from build123d import *

# Parameters (mm, degrees)
SZKIC2_R                   = 1.75
WYTNIJ_WYCI_GNI_CIE1_DEPTH = 15.013168353
SZKIC4_R                   = 3
WYTNIJ_WYCI_GNI_CIE2_DEPTH = 4
SFAZOWANIE1_SIZE           = 1


with BuildPart() as part:
    # Szkic1 → Obrót1 (revolve)
    with BuildSketch(Plane.XY):
        Polygon((-272.858046523, 75.009269975), (-280.358046523, 75.009269975), (-280.358046523, 68.009269975), (-286.871214876, 68.009269975), (-286.871214876, 85.009269975), (-285.871214876, 86.009269975), (-272.858046523, 86.009269975), align=None)
    revolve(axis=Axis((-268.908046523, 1.009269975, 0), (-1, 0, 0)))

    # Szkic2 → Wytnij-wyciągnięcie1 (cut, through all)
    with BuildSketch(Plane.ZY.offset(286.871214876)):
        with Locations((79.5, 1.009269975)):
            Circle(SZKIC2_R)
        with Locations((56.214989104, -55.20571913)):
            Circle(SZKIC2_R)
        with Locations((0, -78.490730025)):
            Circle(SZKIC2_R)
        with Locations((-56.214989104, -55.20571913)):
            Circle(SZKIC2_R)
        with Locations((-79.5, 1.009269975)):
            Circle(SZKIC2_R)
        with Locations((-56.214989104, 57.224259079)):
            Circle(SZKIC2_R)
        with Locations((0, 80.509269975)):
            Circle(SZKIC2_R)
        with Locations((56.214989104, 57.224259079)):
            Circle(SZKIC2_R)
    extrude(amount=-WYTNIJ_WYCI_GNI_CIE1_DEPTH, mode=Mode.SUBTRACT)

    # Szkic4 → Wytnij-wyciągnięcie2 (cut)
    with BuildSketch(Plane.ZY.offset(286.871214876)):
        with Locations((79.5, 1.009269975)):
            Circle(SZKIC4_R)
        with Locations((56.214989104, -55.20571913)):
            Circle(SZKIC4_R)
        with Locations((0, -78.490730025)):
            Circle(SZKIC4_R)
        with Locations((-56.214989104, -55.20571913)):
            Circle(SZKIC4_R)
        with Locations((-79.5, 1.009269975)):
            Circle(SZKIC4_R)
        with Locations((-56.214989104, 57.224259079)):
            Circle(SZKIC4_R)
        with Locations((0, 80.509269975)):
            Circle(SZKIC4_R)
        with Locations((56.214989104, 57.224259079)):
            Circle(SZKIC4_R)
    extrude(amount=-WYTNIJ_WYCI_GNI_CIE2_DEPTH, mode=Mode.SUBTRACT)

    # Sfazowanie1
    sfazowanie1_edges = [part.edges().sort_by_distance(p)[0] for p in [
        (-280.358046523, -65.990730025, 0),
    ]]
    chamfer(sfazowanie1_edges, length=SFAZOWANIE1_SIZE)


solid = part.part
The listing builds one solid part. Answer for the finished solid, in the listing's coordinates (mm). A direction names the side the tool comes from. Give positions to 0.01 mm unless a question says otherwise; leave off trailing zeros.
Item 1: Each of these flat-tipped pins is pushed along its axis until it touches: pin 1 Ø8 at (y, z) = (17, 60) entering from +X; pin 2 Ø5.5 at (y, z) = (57.22, -56.21) entering from +X; pin 3 Ø3 at (y, z) = (-79.5, -1) entering from -X; pin 4 Ø3 at (x, y) = (-276, -41) entering from -Z. Where does it stop, or does it pass through?
Derived:
pin 1: passes through
pin 2: stops at x = -272.86
pin 3: stops at x = -282.87
pin 4: stops at z = -74.73
Item 2: A cutting plane is placed at A-A (x = -275.75). Give the number of separate pieces and of enclosed holes in the cut face, then the cut area to 3 significant figures.
Derived:
separate pieces: 1
enclosed holes: 9
area: 5,420 mm2
Item 3: A tool of negligible diameter and unlimited length cuts with its end or side. For faces 4 (the flat face through (-272.858, 1, 75)), 5 (the cylindrical face through (-284.9, -81.42, -0.65)), 6 (the cylindrical face through (-276.661, -57.715, 45.028)), from which of +Z, -Z, +X, -X, +Y, -Y can it reach the whole face along a straight path? Write none if from no direction.
Derived:
face 4: +Z, -Z, +X, +Y, -Y
face 5: -X
face 6: +X
Item 4: Determine the mould class of faces 1 (the cylindrical face through (-284.899, 54.296, -56.865)), 2 (the cylindrical face through (-279.274, 82.084, -25.532)), 3 (the flat face through (-286.871, 57.4, 36.9)) for opening direction Z: +Z half, -Z half, draft (parallel to the pull), parting line (faces both ways), or undercut.
Derived:
face 1: undercut
face 2: parting line
face 3: draft
Item 5: Find the intervals of material crossed by line 1 along Z through (x, y) = (-283.5, 0); line 2 along Z through (x, y) = (-281, -55); line 3 along Y through (x, z) = (-279.25, 57), in increasing order.
Derived:
line 1: z = -84.99 to -82.33, -76.67 to -66.99, 66.99 to 76.67, 82.33 to 84.99
line 2: z = -63.94 to -57.95, -54.48 to -37.42, 37.42 to 54.48, 57.95 to 63.94
line 3: y = -62.05 to -56.77, -53.64 to -46.18, 48.2 to 55.66, 58.79 to 64.06
